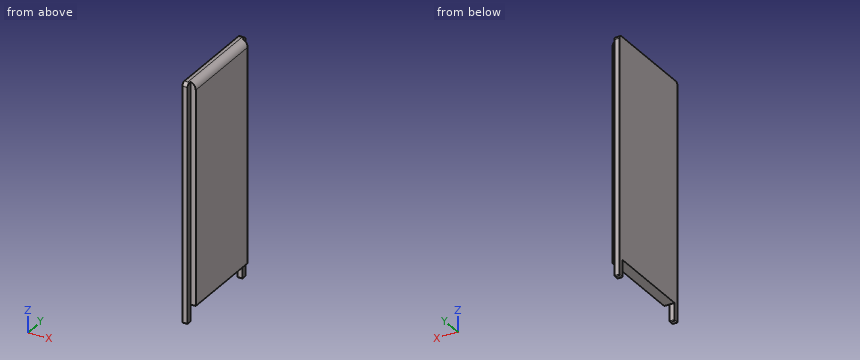
Autodesk Inventor part; units mm, degrees
ref_plane "YZ Plane" through (0, 0, 0) normal (1, 0, 0) x (0, 1, 0)
ref_plane "XZ Plane" through (0, 0, 0) normal (0, 1, 0) x (-1, 0, 0)
ref_plane "XY Plane" through (0, 0, 0) normal (0, 0, 1) x (1, 0, 0)
sketch "Sketch1" plane through (0, 0, 0) normal (0, 0, 1) x (1, 0, 0)
  line L0 (14.9794, -18.4381) -> (14.9794, 9.5619)
  line L1 (16.4794, -16.9381) -> (17.9794, -16.9381)
  line L2 (17.9794, 8.0619) -> (16.4794, 8.0619)
  line L3 (16.4794, 9.5619) -> (16.4794, 8.0619)
  line L4 (16.4794, -16.9381) -> (16.4794, -18.4381)
  line L5 (14.9794, 9.5619) -> (16.4794, 9.5619)
  line L6 (14.9794, -18.4381) -> (16.4794, -18.4381)
  line L7 (16.4794, -16.9381) -> (14.9794, -16.9381)
  line L8 (16.4794, 8.0619) -> (14.9794, 8.0619)
  line L9 (17.9794, 8.0619) -> (17.9794, -16.9381)
  dimension "d3" = 28
  dimension "d4" = 1.5
  dimension "d5" = 1.5
  dimension "d9" = 1.5
  dimension "d10" = 1.5
  dimension "d11" = 3
  dimension "d12" = 1.5
  dimension "d13" = 1.5
extrude "Extrusion1" add sketch "Sketch1" along normal blind 64
extrude "Extrusion2" add sketch "Sketch1" against normal blind 5 contours L0 L7 L4 L6 | L0 L5 L3 L8
fillet "Fillet1" radius 0.25 8 edges at (15.7294, 9.5619, -5) (16.4794, 8.8119, -5) (15.7294, 8.0619, -5) (14.9794, 8.8119, -5) (16.4794, -17.6881, -5) (15.7294, -16.9381, -5) (14.9794, -17.6881, -5) (15.7294, -18.4381, -5)
fillet "Fillet2" radius 1 2 edges at (15.7294, 9.5619, 64) (15.7294, -18.4381, 64)
fillet "Fillet3" radius 2 1 edges at (17.9794, -4.4381, 64)
properties part number "cover"
Geometry check sheet. Reference: the model listing, model coordinates, mm. Round coordinates to 2 decimals unless told otherwise and drop trailing zeros. Order: outer loops, then holes, each group sorted by start corner. A loop starts at its lowest first (then second) coordinate and runs counter-clockwise, first axis right, second up. Notation, with made-up numbers: M -20,53 L 37,53 A35 ccw 37,87 Z; hole C -13,74 d11. An arc over 180 degrees is marked long. Answer in a Markdown table with one row per item.
(1) Sectioned sample at A-A, the plane z = 52. Record the cut outline in (x, y), and give its area (3 significant figures).
Responses:
| item | result |
|---|---|
| outline | M 14.98,-18.44 L 16.48,-18.44 L 16.48,-16.94 L 17.98,-16.94 L 17.98,8.06 L 16.48,8.06 L 16.48,9.56 L 14.98,9.56 Z |
| area | 79.5 mm² |
(2) Sectioned sample at B-B, the plane y = -15. Record the cut outline in (x, z), and give its area (3 significant figures).
Responses:
| item | result |
|---|---|
| outline | M 14.98,0 L 17.98,0 L 17.98,62 A2 ccw 15.98,64 L 14.98,64 Z |
| area | 191 mm² |
(3) Sectioned sample at C-C, the plane x = 17.15. Record the cut outline in (y, z).
Responses:
| item | result |
|---|---|
| outline | M -16.94,0 L 8.06,0 L 8.06,63.62 L -16.94,63.62 Z |
(4) Scan lines: probe 1 along Z at (x, y) = (16, 7); probe 2 along Z at (x, y) = (16.5, -16); probe 3 along Y at (x, z) = (17.7, 20.5). Record each from-to range of solid material in increasing order. Write a range as from..to.
Responses:
| item | result |
|---|---|
| probe 1 | z = 0..64 |
| probe 2 | z = 0..63.93 |
| probe 3 | y = -16.94..8.06 |
(5) Go/stop test with flat-tipped pins: P1, Ø0.9, axis at x = 17, y = -4, coming from the -Z side; P2, Ø0.5, axis at x = 17.5, z = 41.5, coming from the -Y side. Record where each tip stops, or that it passes through.
Responses:
| item | result |
|---|---|
| P1 | stops at z = 0 |
| P2 | stops at y = -16.94 |
